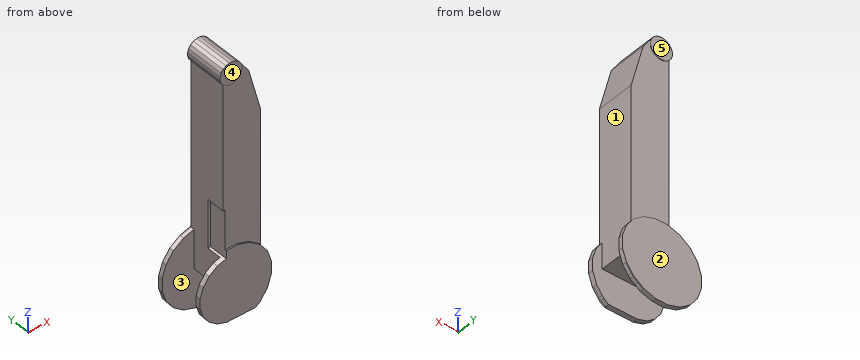
from build123d import *

# Parameters (mm, degrees)
BOSS_EXTRUDE1_DEPTH = 10
BOSS_EXTRUDE2_DEPTH = 90
BOSS_EXTRUDE3_DEPTH = 10
CUT_EXTRUDE1_DEPTH  = 10
CUT_EXTRUDE2_DEPTH  = 90
CUT_EXTRUDE3_DEPTH  = 10
CUT_EXTRUDE4_DEPTH  = 10
CUT_EXTRUDE5_DEPTH  = 10
CUT_EXTRUDE6_DEPTH  = 9.81685291
SKETCH10_W          = 107
SKETCH10_H          = 90
CUT_EXTRUDE7_DEPTH  = 80.18314709
SKETCH11_W          = 6
SKETCH11_H          = 51
CUT_EXTRUDE8_DEPTH  = 134.567114958
BOSS_EXTRUDE4_DEPTH = 4
BOSS_EXTRUDE5_DEPTH = 1
BOSS_EXTRUDE6_DEPTH = 1
BOSS_EXTRUDE7_DEPTH = 2.5
DRAFT1_ANGLE        = 18
CHAMFER1_SIZE       = 6.379377731
CHAMFER1_SIZE2      = 12.134297522


with BuildPart() as part:
    # Sketch1 → Boss-Extrude1 (new body)
    with BuildSketch(Plane(origin=(0, -45, 0), x_dir=(1, 0, 0), z_dir=(0, 1, 0))):
        Polygon((101.03665965, 51.480749424), (85, 73.553317831), (85, 90), (66.671408228, 90), (51.480749424, 101.03665965), (17.739057316, 112), (-17.739057316, 112), (-51.480749424, 101.03665965), (-80.18314709, 80.18314709), (-101.03665965, 51.480749424), (-112, 17.739057316), (-112, -17.739057316), (-101.03665965, -51.480749424), (-80.18314709, -80.18314709), (-51.480749424, -101.03665965), (-22, -110.615535798), (-22, -577.665828314), (-22.193549641, -577.806450359), (-27.96550401, -585.750863999), (-31, -595.09008235), (-31, -604.90991765), (-27.96550401, -614.249136001), (-22.193549641, -622.193549641), (-14.249136001, -627.96550401), (-4.90991765, -631), (4.90991765, -631), (14.249136001, -627.96550401), (22.193549641, -622.193549641), (27.96550401, -614.249136001), (28.064334249, -613.944967802), (51, -581), (85, -455), (85, -73.553317831), (101.03665965, -51.480749424), (112, -17.739057316), (112, 17.739057316), align=None)
    extrude(amount=-BOSS_EXTRUDE1_DEPTH)

    # Sketch2 → Boss-Extrude2 (add)
    with BuildSketch(Plane(origin=(0, -45, 0), x_dir=(-1, 0, 0), z_dir=(0, 1, 0))):
        Polygon((-85, -90), (-85, 455), (-51, 581), (-28.064334249, 613.944967802), (-27.96550401, 614.249136001), (-22.193549641, 622.193549641), (-14.249136001, 627.96550401), (-4.90991765, 631), (4.90991765, 631), (14.249136001, 627.96550401), (22.193549641, 622.193549641), (27.96550401, 614.249136001), (31, 604.90991765), (31, 595.09008235), (27.96550401, 585.750863999), (22.193549641, 577.806450359), (22, 577.665828314), (22, 110.615535798), (51.480749424, 101.03665965), (80.18314709, 80.18314709), (101.03665965, 51.480749424), (112, 17.739057316), (112, -17.739057316), (101.03665965, -51.480749424), (80.18314709, -80.18314709), (51.480749424, -101.03665965), (17.739057316, -112), (-17.739057316, -112), (-51.480749424, -101.03665965), (-66.671408228, -90), align=None)
    extrude(amount=BOSS_EXTRUDE2_DEPTH)

    # Sketch3 → Boss-Extrude3 (add)
    with BuildSketch(Plane(origin=(0, 45, 0), x_dir=(-1, 0, 0), z_dir=(0, 1, 0))):
        Polygon((-85, -73.553317831), (-101.03665965, -51.480749424), (-112, -17.739057316), (-112, 17.739057316), (-101.03665965, 51.480749424), (-85, 73.553317831), (-85, 455), (-51, 581), (-28.064334249, 613.944967802), (-27.96550401, 614.249136001), (-22.193549641, 622.193549641), (-14.249136001, 627.96550401), (-4.90991765, 631), (4.90991765, 631), (14.249136001, 627.96550401), (22.193549641, 622.193549641), (27.96550401, 614.249136001), (31, 604.90991765), (31, 595.09008235), (27.96550401, 585.750863999), (22.193549641, 577.806450359), (22, 577.665828314), (22, 110.615535798), (51.480749424, 101.03665965), (80.18314709, 80.18314709), (101.03665965, 51.480749424), (112, 17.739057316), (112, -17.739057316), (101.03665965, -51.480749424), (80.18314709, -80.18314709), (51.480749424, -101.03665965), (17.739057316, -112), (-17.739057316, -112), (-51.480749424, -101.03665965), (-66.671408228, -90), (-85, -90), align=None)
    extrude(amount=BOSS_EXTRUDE3_DEPTH)

    # Sketch4 → Cut-Extrude1 (cut)
    with BuildSketch(Plane.XZ.offset(55)):
        Polygon((-30.023339436, 89.432885042), (-22, 89.432885042), (-22, 110.615535798), (-51.480749424, 101.03665965), (-80.18314709, 80.18314709), (-101.03665965, 51.480749424), (-112, 17.739057316), (-112, -17.739057316), (-101.03665965, -51.480749424), (-80.18314709, -80.18314709), (-51.480749424, -101.03665965), (-17.739057316, -112), (17.739057316, -112), (51.480749424, -101.03665965), (66.671408228, -90), (-22, -90), (-22, -87.483366864), (-41.368459358, -81.190172933), (-64.432886054, -64.432886054), (-81.190172933, -41.368459358), (-90, -14.254599629), (-90, 14.254599629), (-81.190172933, 41.368459358), (-64.432886054, 64.432886054), align=None)
    extrude(amount=-CUT_EXTRUDE1_DEPTH, mode=Mode.SUBTRACT)

    # Sketch5 → Cut-Extrude2 (cut)
    with BuildSketch(Plane.XZ.offset(45)):
        Polygon((66.671408228, -90), (-22, -90), (-22, 110.615535798), (-51.480749424, 101.03665965), (-80.18314709, 80.18314709), (-101.03665965, 51.480749424), (-112, 17.739057316), (-112, -17.739057316), (-101.03665965, -51.480749424), (-80.18314709, -80.18314709), (-51.480749424, -101.03665965), (-17.739057316, -112), (17.739057316, -112), (51.480749424, -101.03665965), align=None)
    extrude(amount=-CUT_EXTRUDE2_DEPTH, mode=Mode.SUBTRACT)

    # Sketch6 → Cut-Extrude3 (cut)
    with BuildSketch(Plane.XZ.offset(55)):
        Polygon((85, -90), (85, -73.553317831), (73.050785959, -90), align=None)
    extrude(amount=-CUT_EXTRUDE3_DEPTH, mode=Mode.SUBTRACT)

    # Sketch7 → Cut-Extrude4 (cut)
    with BuildSketch(Plane.XZ.offset(55)):
        Polygon((-14.254599629, -90), (-22, -87.483366864), (-22, -90), align=None)
    extrude(amount=-CUT_EXTRUDE4_DEPTH, mode=Mode.SUBTRACT)

    # Sketch8 → Cut-Extrude5 (cut)
    with BuildSketch(Plane(origin=(0, 55, 0), x_dir=(-1, 0, 0), z_dir=(0, 1, 0))):
        Polygon((-80.18314709, -80.18314709), (-85, -73.553317831), (-85, -90), (-66.671408228, -90), align=None)
    extrude(amount=-CUT_EXTRUDE5_DEPTH, mode=Mode.SUBTRACT)

    # Sketch9 → Cut-Extrude6 (cut)
    with BuildSketch(Plane(origin=(0, 0, -90), x_dir=(-1, 0, 0), z_dir=(0, 0, -1))):
        Polygon((-80.18314709, -45), (22, -45), (22, 45), (-80.18314709, 45), (-85, 45), (-85, -45), align=None)
    extrude(amount=-CUT_EXTRUDE6_DEPTH, mode=Mode.SUBTRACT)

    # Sketch10 → Cut-Extrude7 (cut)
    with BuildSketch(Plane(origin=(0, 0, -80.18314709), x_dir=(-1, 0, 0), z_dir=(0, 0, -1))):
        with Locations((-31.5, 0)):
            Rectangle(SKETCH10_W, SKETCH10_H)
    extrude(amount=-CUT_EXTRUDE7_DEPTH, mode=Mode.SUBTRACT)

    # Sketch11 → Cut-Extrude8 (cut)
    with BuildSketch(Plane(origin=(0, 0, 89.432885042), x_dir=(-1, 0, 0), z_dir=(0, 0, -1))):
        with Locations((19, -29.5)):
            Rectangle(SKETCH11_W, SKETCH11_H)
    extrude(amount=-CUT_EXTRUDE8_DEPTH, mode=Mode.SUBTRACT)

    # Sketch12 → Boss-Extrude4 (add)
    with BuildSketch(Plane.XZ.offset(55)):
        Polygon((-16, 89.432885042), (-16, 112), (17.739057316, 112), (51.480749424, 101.03665965), (80.18314709, 80.18314709), (101.03665965, 51.480749424), (112, 17.739057316), (112, -17.739057316), (101.03665965, -51.480749424), (73.050785959, -90), (-14.254599629, -90), (-41.368459358, -81.190172933), (-64.432886054, -64.432886054), (-81.190172933, -41.368459358), (-90, -14.254599629), (-90, 14.254599629), (-81.190172933, 41.368459358), (-64.432886054, 64.432886054), (-30.023339436, 89.432885042), align=None)
    extrude(amount=BOSS_EXTRUDE4_DEPTH)

    # Sketch13 → Boss-Extrude5 (add)
    with BuildSketch(Plane.XZ.offset(55)):
        Polygon((22.193549641, 577.806450359), (14.249136001, 572.03449599), (4.90991765, 569), (-4.90991765, 569), (-14.249136001, 572.03449599), (-22.193549641, 577.806450359), (-27.96550401, 585.750863999), (-31, 595.09008235), (-31, 604.90991765), (-27.96550401, 614.249136001), (-22.193549641, 622.193549641), (-14.249136001, 627.96550401), (-4.90991765, 631), (4.90991765, 631), (14.249136001, 627.96550401), (22.193549641, 622.193549641), (27.96550401, 614.249136001), (31, 604.90991765), (31, 595.09008235), (27.96550401, 585.750863999), align=None)
    extrude(amount=BOSS_EXTRUDE5_DEPTH)

    # Sketch14 → Boss-Extrude6 (add)
    with BuildSketch(Plane(origin=(0, 55, 0), x_dir=(-1, 0, 0), z_dir=(0, 1, 0))):
        Polygon((-14.249136001, 572.03449599), (-22.193549641, 577.806450359), (-27.96550401, 585.750863999), (-31, 595.09008235), (-31, 604.90991765), (-27.96550401, 614.249136001), (-22.193549641, 622.193549641), (-14.249136001, 627.96550401), (-4.90991765, 631), (4.90991765, 631), (14.249136001, 627.96550401), (22.193549641, 622.193549641), (27.96550401, 614.249136001), (31, 604.90991765), (31, 595.09008235), (27.96550401, 585.750863999), (22.193549641, 577.806450359), (14.249136001, 572.03449599), (4.90991765, 569), (-4.90991765, 569), align=None)
    extrude(amount=BOSS_EXTRUDE6_DEPTH)

    # Sketch15 → Boss-Extrude7 (add)
    with BuildSketch(Plane(origin=(0, 55, 0), x_dir=(-1, 0, 0), z_dir=(0, 1, 0))):
        Polygon((-80.18314709, -80.18314709), (-101.03665965, -51.480749424), (-112, -17.739057316), (-112, 17.739057316), (-101.03665965, 51.480749424), (-80.18314709, 80.18314709), (-51.480749424, 101.03665965), (-17.739057316, 112), (17.739057316, 112), (51.480749424, 101.03665965), (80.18314709, 80.18314709), (101.03665965, 51.480749424), (112, 17.739057316), (112, -17.739057316), (101.03665965, -51.480749424), (80.18314709, -80.18314709), (51.480749424, -101.03665965), (17.739057316, -112), (-17.739057316, -112), (-51.480749424, -101.03665965), align=None)
    extrude(amount=BOSS_EXTRUDE7_DEPTH)

    # Draft1
    draft1_faces = [part.faces().sort_by_distance(p)[0] for p in [
        (-20.780579815, -36.705876441, 89.432885042),
    ]]
    draft(draft1_faces, Plane(origin=(-16, -4, 224), x_dir=(0, 0, -1), z_dir=(-1, 0, 0)), DRAFT1_ANGLE)

    # Chamfer1
    chamfer1_edges = [part.edges().sort_by_distance(p)[0] for p in [
        (73.050785959, -52, -90),
    ]]
    chamfer1_side = [part.faces().sort_by_distance(p)[0] for p in [
        (29.398093165, -52, -90),
    ]]
    chamfer(chamfer1_edges, length=CHAMFER1_SIZE, length2=CHAMFER1_SIZE2, reference=chamfer1_side[0])


solid = part.part
Build history of the part. All positions in model axes, mm. Face numbers are marked on the shaded views. A direction names the side the tool comes from. Coordinates: 2 decimals unless noted, no trailing zeros. Order: outer loops, then holes, each group sorted by start corner. A loop starts at its lowest first (then second) coordinate and runs counter-clockwise, first axis right, second up. Notation, with made-up numbers: (12, 81) - (61, 81) arc R24 cw to (61, 101) - close; hole circle Ø8 at (84, 28). An arc over 180 degrees is marked (long way). Put each result on its own line as item: value.
1. Saw through at C-C (y = -20). Write the cut outline in (x, z), and give its area (3 significant figures).
Answer sheet:
outline: (-31, 595.09) - (-27.97, 585.75) - (-22.19, 577.81) - (-22, 577.67) - (-22, 224) - (-16, 224) - (-16, 89.43) - (-22, 87.48) - (-22, 0) - (85, 0) - (85, 455) - (51, 581) - (28.06, 613.94) - (27.97, 614.25) - (22.19, 622.19) - (14.25, 627.97) - (4.91, 631) - (-4.91, 631) - (-14.25, 627.97) - (-22.19, 622.19) - (-27.97, 614.25) - (-31, 604.91) - close
area: 62,200 mm^2
2. Drop flat-ended pins along their axis: P1, Ø2, axis at x = 71.5, y = -4.5, coming from the -Z side; P2, Ø0.5, axis at y = 55.5, z = 598.5, coming from the +X side; P3, Ø5, axis at x = 26.5, y = -13.5, coming from the +Z side. Give the stop position or say it passes through.
Answer sheet:
P1: stops at z = 0
P2: stops at x = 31
P3: stops at z = 619.71
3. Saw through at D-D (z = 143). Write the cut outline in (x, y).
Answer sheet:
outline: (-22, -4) - (-16, -4) - (-16, -55) - (85, -55) - (85, 55) - (-22, 55) - close
4. Saw through at B-B (z = 26). Write the cut outline in (x, y).
Answer sheet:
outline: (-109.32, 45) - (-22, 45) - (-22, -45) - (-86.18, -45) - (-86.18, -59) - (109.32, -59) - (109.32, -45) - (85, -45) - (85, 45) - (109.32, 45) - (109.32, 57.5) - (-109.32, 57.5) - close
5. Saw through at A-A (y = 9). Write the cut outline in (x, z), and give its area (3 significant figures).
Answer sheet:
outline: (-31, 595.09) - (-27.97, 585.75) - (-22.19, 577.81) - (-22, 577.67) - (-22, 0) - (85, 0) - (85, 455) - (51, 581) - (28.06, 613.94) - (27.97, 614.25) - (22.19, 622.19) - (14.25, 627.97) - (4.91, 631) - (-4.91, 631) - (-14.25, 627.97) - (-22.19, 622.19) - (-27.97, 614.25) - (-31, 604.91) - close
area: 63,000 mm^2
6. Tool access for the marked faces 1 and 2: list every direction of +Z, -Z, +X, -X, +Y, -Y with a clear straight run to the whole face (end or side of a thin tool).
Answer sheet:
face 1: +Z, +X
face 2: +Z, -Z, +X, -X, +Y
7. Probe line 1 along Z through (x, y) = (3.5, 43); line 2 along X through (y, z) = (26.5, 103); line 3 along Y through (x, z) = (63.5, 387.5). List the from-to ranges inside material, lowest first. Write a range as [from, to].
Answer sheet:
line 1: z = [0, 631]
line 2: x = [-22, 85]
line 3: y = [-55, 55]
8. Pull direction Y, two halves, no side cores. Call the marked faces 3, 4 and 5: pulls with the +Y half, pulls with the -Y half, needs draft (parallel to the pull), parting line crosses it, or undercut.
Answer sheet:
face 3: undercut
face 4: pulls with the -Y half
face 5: pulls with the +Y half
